Autodesk Inventor part; units mm, degrees
ref_plane "Work Plane1" through (-15, 15, 7) normal (0, 0, 1) x (1, 0, 0)
ref_plane "Work Plane2" through (15, 7, 19.5) normal (0, 0, -1) x (-1, 0, 0)
ref_plane "YZ Plane" through (0, 0, 0) normal (1, 0, 0) x (0, 1, 0)
sketch "Sketch1" plane through (0, 0, 0) normal (0, 0, 1) x (1, 0, 0)
  line L0 (0, 0) -> (-75, 0)
  line L1 (0, 0) -> (0, 50)
  line L2 (0, 50) -> (-38, 50)
  line L3 (-75, 0) -> (-75, 5)
  spline S0 degree 3 poles (-38, 50) (-46.7224, 6.6996) (-125.1064, 18.5226) (-28.5296, -55.0422) knots 0 0 0 0 1 1 1 1
  point P0 (-58.1914, 22.009)
  dimension "d0" = 75
  dimension "d1" = 50
  dimension "d2" = 38
  dimension "d3" = 5
revolve "Revolution1" add sketch "Sketch1" angle 360 about axis through (0, 0, 0) along (0, 1, 0)
sketch "Sketch2" plane through (0, 50, 0) normal (0, 1, 0) x (1, 0, 0)
  line L0 (-15, 24) -> (15, 24)
  line L1 (15, 24) -> (15, -24)
  line L2 (15, -24) -> (-15, -24)
  line L3 (-15, -24) -> (-15, 24)
  point P0 (0, 0)
  dimension "d5" = 30
  dimension "d6" = 48
  dimension "d7" = 24
  dimension "d8" = 15
extrude "Extrusion1" cut sketch "Sketch2" against normal blind 35
sketch "Sketch3" plane through (0, 15, 0) normal (0, 1, 0) x (1, 0, 0)
  line L0 (15, -24) -> (-15, -24)
  line L1 (-15, -24) -> (-15, 24)
  line L2 (15, -24) -> (-15, -24)
  line L3 (-15, -24) -> (-15, -7)
  line L4 (-15, -7) -> (15, -7)
  line L5 (15, -7) -> (15, -24)
  point P0 (0, 0)
  dimension "d11" = 17
extrude "Extrusion2" cut sketch "Sketch3" against normal blind 8
sketch "Sketch4" plane through (0, 0, 0) normal (0, 0, 1) x (1, 0, 0)
  circle A0 centre (-26, 38) radius 2.6
  circle A1 centre (-53, 12) radius 2.6
  line L0 (75, 0) -> (-75, 0)
  line L1 (38, 50) -> (-38, 50)
  line L2 (-75, 0) -> (-75, 5)
  line L3 (15, 50) -> (-15, 50) construction
  line L4 (0, 50) -> (0, 20.8019) construction
  circle A2 centre (26, 38) radius 2.6
  circle A3 centre (53, 12) radius 2.6
  point P0 (0, 0)
  dimension "d14" = 5.2
  dimension "d15" = 5.2
  dimension "d16" = 12
  dimension "d17" = 12
  dimension "d18" = 22
  dimension "d19" = 12
extrude "Extrusion3" cut sketch "Sketch4" along normal blind 52 and the other way blind 52
ref_plane "Work Plane1" through (-15, 15, 7) normal (0, 0, 1) x (1, 0, 0)
split "Split1" plane through (-15, 15, 7) removes the side toward (0, 0, -1)
sketch "Sketch6" plane through (0, 0, 0) normal (0, -1, 0) x (1, 0, 0)
  circle A0 centre (0, 0) radius 10.5
  dimension "d25" = 21
extrude "Extrusion4" cut sketch "Sketch6" against normal blind 2.5
ref_plane "Work Plane2" through (15, 7, 19.5) normal (0, 0, -1) x (-1, 0, 0)
sketch "Sketch7" plane through (15, 7, 19.5) normal (0, 0, -1) x (-1, 0, 0)
  circle A0 centre (41, 31) radius 2.6
  circle A1 centre (41, 31) radius 6.25
  circle A2 centre (-11, 31) radius 2.6
  circle A3 centre (-11, 31) radius 6.25
  circle A4 centre (-38, 5) radius 2.6
  circle A5 centre (-38, 5) radius 6.25
  circle A6 centre (68, 5) radius 2.6
  circle A7 centre (68, 5) radius 6.25
  point P0 (15, -7)
  dimension "d29" = 12.5
  dimension "d30" = 12.5
  dimension "d31" = 12.5
  dimension "d32" = 12.5
extrude "Extrusion5" cut sketch "Sketch7" against normal blind 50 contours A0 | A1 | A2 | A3 | A4 | A5 | A6 | A7
properties part number "Podstawa 01-1"
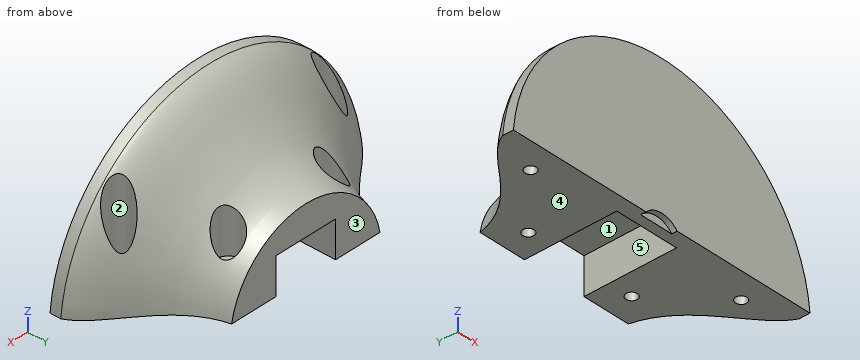
Design review of the part built by this model. Coordinates are the model's own, in mm. Face numbers are marked on the shaded views. A direction names the side the tool comes from. Coordinates: 2 decimals unless noted, no trailing zeros. Use one line per item in the form item = value.
Q1. Insertion check: pin 1 Ø4.5 at (x, y) = (-53, 12) entering from -Z (1 decimal); pin 2 Ø8 at (x, z) = (32, 40) entering from +Y (3 decimals); pin 3 Ø8.5 at (y, z) = (18.5, 13) entering from -X; pin 4 Ø8 at (x, y) = (5.5, 30) entering from -Z. Each pin has a flat end and moves straight along its axis. Give the tip position at first contact, or say it passes through.
Taken from the geometry:
pin_1 = through
pin_2 = 32.075
pin_3 = -66.49
pin_4 = 24
Q2. For probe 1 along X at (y, z) = (38, 16.5); probe 2 along X at (y, z) = (38, 17.25); probe 3 along Y at (x, z) = (-26, 13), list the stretches that pass through material, from the lowest coordinate up.
Taken from the geometry:
probe_1 = -39.47 to -28.6, -23.4 to -15, 15 to 23.4, 28.6 to 39.47
probe_2 = -39.15 to -28.6, -23.4 to -15, 15 to 23.4, 28.6 to 39.15
probe_3 = 0 to 35.4, 40.6 to 50
Q3. The part is to be moulded in two halves that separate along X. For the marked faces 4 and 5, say which applies: +X half, -X half, draft (parallel to the pull), parting line (faces both ways), or undercut.
Taken from the geometry:
face_4 = draft
face_5 = undercut
Q4. Machinability: for the marked faces 1, 2 and 3, which of the approach directions +Z, -Z, +X, -X, +Y, -Y give a long, thin tool a straight path to every point of the face, cutting with its end or side? Answer none if there is none.
Taken from the geometry:
face_1 = -Z, +Y
face_2 = +Z
face_3 = +Z, -Z, +X, -X, +Y
Q5. Consider section A-A (y = 12). Count the separate pieces of the cut face and the enclosed holes in it, plus the area to 3 significant figures.
Taken from the geometry:
separate_pieces = 3
enclosed_holes = 0
area = 5,440 mm^2
